Source: three-view drawing plus pictorial views. Frame: mm from the lowest corner of the part. Give positions to 0.01 mm unless a question says otherwise; leave off trailing zeros. Order: outer loops, then holes, each group sorted by start corner. A loop starts at its lowest first (then second) coordinate and runs counter-clockwise, first axis right, second up. Notation, with made-up numbers: (10.5, -31.5) -> (43.5, -31.5) arc R20 ccw to (43.5, 2.5) -> close; hole circle Ø10 at (-14, -3). An arc over 180 degrees is marked (long way). One line per question, with ' | ' between items.
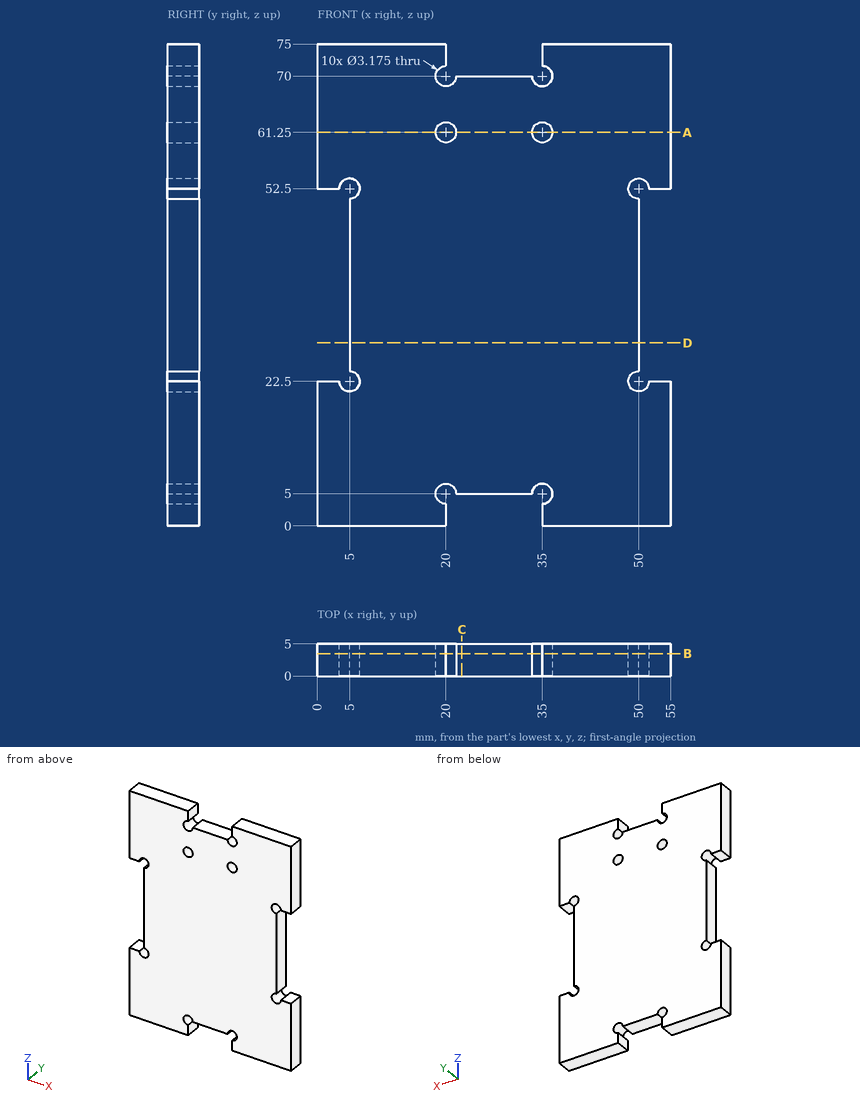
1) Section A-A on z = 61.25. Return loops of the section in (x, y).
Check result:
outline: (0, 0) -> (18.41, 0) -> (18.41, 5) -> (0, 5) -> close; (21.59, 0) -> (33.41, 0) -> (33.41, 5) -> (21.59, 5) -> close; (36.59, 0) -> (55, 0) -> (55, 5) -> (36.59, 5) -> close
2) Contact query for flat-ended pins moving along their axis: pin 1 Ø2.5 at (y, z) = (3.5, 36) entering from +X; pin 2 Ø2 at (y, z) = (2.5, 36.5) entering from -X; pin 3 Ø2.5 at (x, y) = (29, 1.5) entering from +Z. Output: stop coordinate, or through.
Check result:
pin 1: stops at x = 50 | pin 2: stops at x = 5 | pin 3: stops at z = 70
3) Section B-B on y = 3.5. Count the separate pieces of the cut face and the enclosed holes in it, plus the area to 3 significant figures.
Check result:
separate pieces: 1 | enclosed holes: 2 | area: 3,610 mm^2
4) Section D-D on z = 28.5. Return loops of the section in (x, y).
Check result:
outline: (5, 0) -> (50, 0) -> (50, 5) -> (5, 5) -> close
5) Material intervals for probe 1 along X at (y, z) = (0.75, 3); probe 2 along Z at (x, y) = (33, 1.25); probe 3 along Z at (x, y) = (49.5, 1.05), sorted ascending. Write a range as from..to.
Check result:
probe 1: x = 0..20, 35..55 | probe 2: z = 5..70 | probe 3: z = 0..20.99, 24.01..50.99, 54.01..75
6) Section C-C on x = 22.5. Return loops of the section in (y, z), plus the area to 3 significant figures.
Check result:
outline: (0, 5) -> (5, 5) -> (5, 70) -> (0, 70) -> close | area: 325 mm^2
